The model under review builds one solid part; all positions refer to its coordinate system, in mm. Give positions to 0.01 mm unless a question says otherwise; leave off trailing zeros. Loops run counter-clockwise (first coordinate to the right, second up) from the corner with the lowest first, then second, coordinate; pieces in that order, holes last. Notation, with made-up numbers: M 54.5,21.25 L 101.5,21.25 A16 cw 101.5,40.25 Z; hole C 31,-19.75 d5. An arc over 180 degrees is marked long. Return JSON: item names as keys, results as strings. Group by question number.
```python
from build123d import *

# Parameters (mm, degrees)
F0_R     = 3.96875
F1_DEPTH = 1


with BuildPart() as f1:
    # F0 (on Front) → F1 (new body)
    with BuildSketch(Plane.XZ):
        with BuildLine():
            Line((8.509, 9.525), (0, 9.525))
            Line((0, 9.525), (-8.509, 9.525))
            ThreePointArc((-8.509, 9.525), (-9.22742, 9.22742), (-9.525, 8.509))
            Line((-9.525, 8.509), (-9.525, -21.209))
            ThreePointArc((-9.525, -21.209), (-9.017, -21.717), (-9.525, -22.225))
            Line((-9.525, -22.225), (-9.525, -46.609))
            ThreePointArc((-9.525, -46.609), (-9.22742, -47.32742), (-8.509, -47.625))
            Line((-8.509, -47.625), (0, -47.625))
            Line((0, -47.625), (8.001, -47.625))
            ThreePointArc((8.001, -47.625), (8.71942, -47.32742), (9.017, -46.609))
            Line((9.017, -46.609), (9.017, -41.783))
            ThreePointArc((9.017, -41.783), (8.547669, -41.080597), (9.37621, -40.91579))
            Line((9.37621, -40.91579), (26.33258, -23.95942))
            ThreePointArc((26.33258, -23.95942), (26.552821, -22.852194), (25.614159, -22.225))
            Line((25.614159, -22.225), (9.525, -22.225))
            ThreePointArc((9.525, -22.225), (8.65779, -22.58421), (9.017, -21.717))
            ThreePointArc((9.017, -21.717), (9.16579, -21.35779), (9.525, -21.209))
            Line((9.525, -21.209), (9.525, 8.509))
            ThreePointArc((9.525, 8.509), (9.22742, 9.22742), (8.509, 9.525))
        make_face()
        Circle(F0_R, mode=Mode.SUBTRACT)
    extrude(amount=F1_DEPTH)


solid = f1.part
```
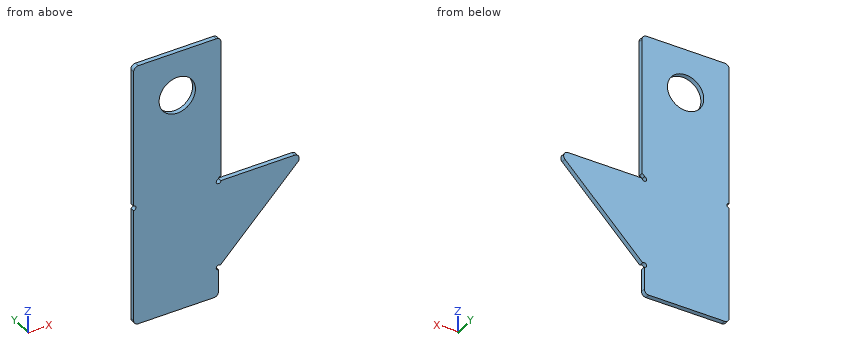
(1) For pin 1 (0.5 mm diameter, centred on y = -0.5, z = -13, fed in from +X) (3 decimals), flat-tipped, find the tip position at first contact; note if it passes through.
(2) Add section A-A (x = 0). Write out the cut boundary in (y, z) (3 decimals).
(3) Add section D-D (z = -13.5). Write out the cut boundary in (x, y) (3 decimals), and give its area (4 significant figures).
(4) For probe 1 along Z at (x, y) = (0, -0.15) (3 decimals); probe 2 along X at (y, z) = (-0.05, -12.5) (3 decimals); probe 3 along Z at (x, y) = (1, -0.3) (3 decimals), list the stretches that pass through material, from the lowest coordinate up.
(5) Add section C-C (y = -0.55). Write out the cut boundary in (x, z) (1 decimal).
(6) Add section B-B (z = 0). Write out the cut boundary in (x, y) (3 decimals).
Verdict:
{
 "1": {"pin 1": "stops at x = 9.525"},
 "2": {"outline": "M -1,-47.625 L 0,-47.625 L 0,-3.969 L -1,-3.969 Z; M -1,3.969 L 0,3.969 L 0,9.525 L -1,9.525 Z"},
 "3": {"outline": "M -9.525,-1 L 9.525,-1 L 9.525,0 L -9.525,0 Z", "area": "19.05 mm²"},
 "4": {"probe 1": "z = -47.625 to -3.969, 3.969 to 9.525", "probe 2": "x = -9.525 to 9.525", "probe 3": "z = -47.625 to -3.841, 3.841 to 9.525"},
 "5": {"outline": "M -9.5,-46.6 A1 ccw -8.5,-47.6 L 8,-47.6 A1 ccw 9,-46.6 L 9,-41.8 A0.5 cw long 9.4,-40.9 L 26.3,-24 A1 ccw 25.6,-22.2 L 9.5,-22.2 A0.5 cw long 9,-21.7 A0.5 cw 9.5,-21.2 L 9.5,8.5 A1 ccw 8.5,9.5 L -8.5,9.5 A1 ccw -9.5,8.5 L -9.5,-21.2 A0.5 cw -9.5,-22.2 Z; hole C 0,0 d7.9"},
 "6": {"outline": "M -9.525,-1 L -3.969,-1 L -3.969,0 L -9.525,0 Z; M 3.969,-1 L 9.525,-1 L 9.525,0 L 3.969,0 Z"}
}
